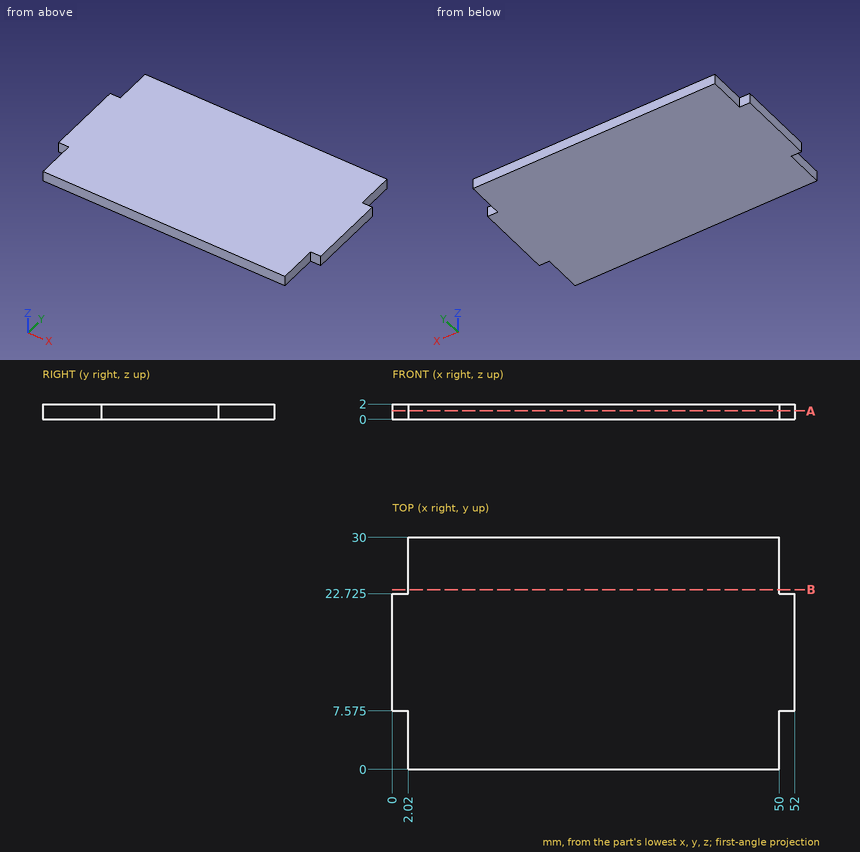
Print and shaded views of the part. All mm, measured from the part's lowest x, y and z. Coordinates: 2 decimals unless noted, no trailing zeros. Order: outer loops, then holes, each group sorted by start corner. A loop starts at its lowest first (then second) coordinate and runs counter-clockwise, first axis right, second up. Notation, with made-up numbers: (26, 12) -> (45, 12) arc R20 ccw to (45, 34) -> close; hole circle Ø8 at (-33.75, 45). An arc over 180 degrees is marked (long way). Answer as a JSON object with one key per item and string values. Group by question number.
1) Flat gauge pins, fed straight in: pin 1 (1 mm diameter, centred on y = 3, z = 0.5, fed in from +X); pin 2 (0.6 mm diameter, centred on x = 1, z = 1, fed in from -Y) (3 decimals); pin 3 (12 mm diameter, centred on x = 30, y = 16, fed in from -Z); pin 4 (1 mm diameter, centred on x = 1, z = 0.5, fed in from +Y) (3 decimals). Where does each tip first touch, or does it go through?
2) Drill centre line: L1, parallel to X at y = 23, z = 0.35. Where is it in solid material? Low to high.
3) Cut at A-A, the plane z = 1.1. Write the cut outline in (x, y) (3 decimals), then the cut area to 3 significant figures.
4) Cut at B-B, the plane y = 23.25. Write the cut outline in (x, z).
Check values:
{
 "1": {"pin 1": "stops at x = 50", "pin 2": "stops at y = 7.575", "pin 3": "stops at z = 0", "pin 4": "stops at y = 22.725"},
 "2": {"L1": "x = 2.02 to 50"},
 "3": {"outline": "(0, 7.575) -> (2.02, 7.575) -> (2.02, 0) -> (50, 0) -> (50, 7.575) -> (52, 7.575) -> (52, 22.725) -> (50, 22.725) -> (50, 30) -> (2.02, 30) -> (2.02, 22.725) -> (0, 22.725) -> close", "area": "1,500 mm²"},
 "4": {"outline": "(2.02, 0) -> (50, 0) -> (50, 2) -> (2.02, 2) -> close"}
}
